```python
from build123d import *

# Parameters (mm, degrees)
SKETCH1_W                       = 50
SKETCH1_H                       = 5
BOSS_EXTRUDE1_DEPTH             = 24
SKETCH5_W                       = 76
SKETCH5_H                       = 20
BOSS_EXTRUDE3_DEPTH             = 8
BOSS_EXTRUDE4_REACH             = 54.953
BOSS_EXTRUDE4_DIRECTION_2_REACH = 54.953
CUT_EXTRUDE4_DEPTH              = 50.839743178
FILLET1_R                       = 4
SKETCH8_R                       = 1.55
CUT_EXTRUDE5_DEPTH              = 85.474848328
BOSS_EXTRUDE2_REACH             = 54.953
SKETCH4_R                       = 7.5
CUT_EXTRUDE3_DEPTH              = 56.145262716


with BuildPart() as part:
    # Sketch1 → Boss-Extrude1 (new body)
    with BuildSketch(Plane(origin=(0, 0, 0), x_dir=(1, 0, 0), z_dir=(0, 1, 0))):
        Rectangle(SKETCH1_W, SKETCH1_H)
    extrude(amount=BOSS_EXTRUDE1_DEPTH)


with BuildPart() as body_2:
    # Sketch5 → Boss-Extrude3 (new body)
    with BuildSketch(Plane(origin=(0, 0, 0), x_dir=(1, 0, 0), z_dir=(0, 1, 0))):
        with Locations((0, -18)):
            Rectangle(SKETCH5_W, SKETCH5_H)
    extrude(amount=BOSS_EXTRUDE3_DEPTH)

    # Boss-Extrude4: up to this face of the body (flat: up to its plane)
    boss_extrude4_end = Plane(body_2.part.faces().sort_by_distance((38, 4, 18))[0])
    # Sketch6 → Boss-Extrude4 (add, up to the picked face)
    with BuildSketch(Plane(origin=(0, 0, 0), x_dir=(0, 0, -1), z_dir=(1, 0, 0)), mode=Mode.PRIVATE) as boss_extrude4_sk1:
        Polygon((-11.313708499, 8), (0, 19.313708499), (2.5, 19.313708499), (2.5, 0), (-11.313708499, 0), align=None)
    boss_extrude4_tool1 = split(extrude(boss_extrude4_sk1.sketch, amount=BOSS_EXTRUDE4_REACH, mode=Mode.PRIVATE), bisect_by=boss_extrude4_end, keep=Keep.BOTH, mode=Mode.PRIVATE)

    add(part.part)  # Boss-Extrude4 merges part
    add(boss_extrude4_tool1.solids().sort_by(Axis((0, 7.799404, 3.417281), (1, 0, 0)))[0])

    # Boss-Extrude4 direction 2: up to this face of the body (flat: up to its plane)
    boss_extrude4_direction_2_end = Plane(body_2.part.faces().sort_by_distance((-38, 4, 18))[0])
    # Sketch6 → Boss-Extrude4 direction 2 (add, up to the picked face)
    with BuildSketch(Plane(origin=(0, 0, 0), x_dir=(0, 0, -1), z_dir=(1, 0, 0)), mode=Mode.PRIVATE) as boss_extrude4_direction_2_sk1:
        Polygon((-11.313708499, 8), (0, 19.313708499), (2.5, 19.313708499), (2.5, 0), (-11.313708499, 0), align=None)
    boss_extrude4_direction_2_tool1 = split(extrude(boss_extrude4_direction_2_sk1.sketch, amount=-BOSS_EXTRUDE4_DIRECTION_2_REACH, mode=Mode.PRIVATE), bisect_by=boss_extrude4_direction_2_end, keep=Keep.BOTH, mode=Mode.PRIVATE)
    add(boss_extrude4_direction_2_tool1.solids().sort_by(Axis((0, 7.799404, 3.417281), (-1, 0, 0)))[0])

    # Sketch7 → Cut-Extrude4 (cut, symmetric)
    with BuildSketch(Plane(origin=(0, 8, 0), x_dir=(1, 0, 0), z_dir=(0, 1, 0))):
        with BuildLine():
            Line((-12, -17.5), (-12, -28))
            Line((-12, -28), (12, -28))
            Line((12, -28), (12, -17.5))
            ThreePointArc((12, -17.5), (0, -5.5), (-12, -17.5))
        make_face()
        with BuildLine():
            Line((-31.5, -16.5), (-31.5, -28))
            Line((-31.5, -28), (-18.5, -28))
            Line((-18.5, -28), (-18.5, -16.5))
            ThreePointArc((-18.5, -16.5), (-25, -10), (-31.5, -16.5))
        make_face()
    cut_extrude4 = extrude(amount=CUT_EXTRUDE4_DEPTH, both=True, mode=Mode.SUBTRACT)

    # Mirror2: Cut-Extrude4 across plane
    add(cut_extrude4.mirror(Plane(origin=(0, 0, 0), x_dir=(0, 0, 1), z_dir=(1, 0, 0))), mode=Mode.SUBTRACT)

    # Fillet1
    fillet1_edges = [body_2.edges().sort_by_distance(p)[0] for p in [
        (-34.75, 0, 28),
        (-34.75, 8, 28),
        (34.75, 0, 28),
        (34.75, 8, 28),
        (15.25, 8, 28),
        (15.25, 0, 28),
        (-15.25, 0, 28),
        (-15.25, 8, 28),
    ]]
    fillet(fillet1_edges, radius=FILLET1_R - 0.0001)  # a hair under: the kernel refuses the full size

    # Sketch8 → Cut-Extrude5 (cut, through all)
    with BuildSketch(Plane(origin=(38, 0, 0), x_dir=(0, 0, -1), z_dir=(1, 0, 0))):
        with Locations((-24, 4)):
            Circle(SKETCH8_R)
    extrude(amount=-CUT_EXTRUDE5_DEPTH, mode=Mode.SUBTRACT)

    # Boss-Extrude2: up to this face of the body (flat: up to its plane)
    boss_extrude2_end = Plane(body_2.part.faces().sort_by_distance((0, 24, 0))[0])
    # Sketch2 → Boss-Extrude2 (add, up to the picked face)
    with BuildSketch(Plane(origin=(0, 0, 0), x_dir=(1, 0, 0), z_dir=(0, 1, 0)), mode=Mode.PRIVATE) as boss_extrude2_sk1:
        with BuildLine():
            Line((19, 5.6), (41, 5.6))
            ThreePointArc((41, 5.6), (30, -5.4), (19, 5.6))
        make_face()
    boss_extrude2_tool1 = split(extrude(boss_extrude2_sk1.sketch, amount=BOSS_EXTRUDE2_REACH, mode=Mode.PRIVATE), bisect_by=boss_extrude2_end, keep=Keep.BOTH, mode=Mode.PRIVATE)
    boss_extrude2 = boss_extrude2_tool1.solids().sort_by(Axis((30, 0, -0.931455), (0, 1, 0)))[0]
    add(boss_extrude2)

    # Sketch4 → Cut-Extrude3 (cut, through all)
    with BuildSketch(Plane(origin=(0, 0, 0), x_dir=(1, 0, 0), z_dir=(0, 1, 0))):
        with Locations((30, 5.6)):
            Circle(SKETCH4_R)
    cut_extrude3 = extrude(amount=CUT_EXTRUDE3_DEPTH, mode=Mode.SUBTRACT)

    # Mirror1: Boss-Extrude2, Cut-Extrude3 across plane
    add(boss_extrude2.mirror(Plane(origin=(0, 0, 0), x_dir=(0, 0, 1), z_dir=(1, 0, 0))))
    add(cut_extrude3.mirror(Plane(origin=(0, 0, 0), x_dir=(0, 0, 1), z_dir=(1, 0, 0))), mode=Mode.SUBTRACT)


solid = body_2.part
```
For this review, take the finished solid that the model builds, in its own axes (mm). A direction names the side the tool comes from. Give positions to 0.01 mm unless a question says otherwise; leave off trailing zeros. Loops run counter-clockwise (first coordinate to the right, second up) from the corner with the lowest first, then second, coordinate; pieces in that order, holes last. Notation, with made-up numbers: M -35.5,13 L 23.5,13 A26 cw 23.5,44 Z; hole C 71.25,15 d3. An arc over 180 degrees is marked long. One line per item, written item: value. Start each with the question number.
Q1. Add section C-C (y = 19.5). Give the boundary of the cut face in (x, z), and give its area (3 significant figures).
Q2. Add section B-B (x = 0). Give the boundary of the cut face in (y, z), and give its area (3 significant figures).
Q3. Add section D-D (z = 1). Give the boundary of the cut face in (x, y).
Q4. Draft analysis for pull direction Z (two halves, no side actions). For faces 6 (the face through (-29.84, 11.83, 1.9)), 7 (the face through (38, 5, 12)), 8 (the face through (34.796, 3.406, 22.568)), state which applies: released by +Z, released by -Z, zero draft, split by the parting line, or undercut.
Q5. Machinability: for faces 1 (the face through (-35, 8, 18)), 2 (the face through (0.532, 14.697, 4.616)), 3 (the face through (29.84, 11.83, 1.9)), 4 (the face through (31.5, 4, 22)), 5 (the face through (-39, 12, -5.6)), which of the approach directions +Z, -Z, +X, -X, +Y, -Y give a long, thin tool a straight path to every point of the face, cutting with its end or side? Answer none if there is none.
Q6. Clearance check with flat-ended pins moving along their axes: pin 1 Ø9 at (y, z) = (3, 23) entering from +X; pin 2 Ø5 at (y, z) = (9, 10) entering from -X; pin 3 Ø5.5 at (x, z) = (18, 15) entering from +Y. State where each tip first meets the part, or that it passes through.
Q7. For L1, parallel to X at y = 2, z = 23; L2, parallel to Y at x = 36, z = 24; L3, parallel to X at y = 12, z = -3.5, list the stretches that pass through material, from the lowest coordinate up.
Q8. Add section A-A (z = 6.5). Give the boundary of the cut face in (x, y), and give its area (3 significant figures).
Reply:
1. outline: M -41,-5.6 L -37.5,-5.6 A7.5 cw -22.5,-5.6 L -19,-5.6 A11 ccw -19.45,-2.5 L 19.45,-2.5 A11 ccw 19,-5.6 L 22.5,-5.6 A7.5 cw 37.5,-5.6 L 41,-5.6 A11 ccw 22.56,2.5 L -22.56,2.5 A11 ccw Z
1. area: 410 mm²
2. outline: M 0,-2.5 L 24,-2.5 L 24,2.5 L 16.81,2.5 L 13.81,5.5 L 0,5.5 Z
2. area: 166 mm²
3. outline: M -38.8,0 L -33.56,0 L -33.56,24 L -38.8,24 Z; M -26.44,0 L 26.44,0 L 26.44,24 L -26.44,24 Z; M 33.56,0 L 38.8,0 L 38.8,24 L 33.56,24 Z
4. face 6: released by -Z
4. face 7: zero draft
4. face 8: undercut
5. face 1: +Z, +X, -X, +Y
5. face 2: +Z, +Y
5. face 3: -Z, +Y, -Y
5. face 4: +Z, +Y, -Y
5. face 5: -Z, +X, -X, +Y, -Y
6. pin 1: x = 38
6. pin 2: x = -38
6. pin 3: y = 8
7. L1: -38 to -31.5, -18.5 to -12, 12 to 18.5, 31.5 to 38
7. L2: 0 to 2.45, 5.55 to 8
7. L3: -40.8 to -37.2, -22.8 to -19.2, 19.2 to 22.8, 37.2 to 40.8
8. outline: M -38,0 L -4.8,0 L -4.8,12.81 L -38,12.81 Z; M 4.8,0 L 38,0 L 38,12.81 L 4.8,12.81 Z
8. area: 851 mm²
